Input: part model. Units: mm. Frame: model coordinates. A direction names the side the tool comes from. Give positions to 0.01 mm unless a question says otherwise; leave off trailing zeros. Loops run counter-clockwise (first coordinate to the right, second up) from the corner with the lowest first, then second, coordinate; pieces in that order, holes last. Notation, with made-up numbers: (-11, -34.5) - (44, -34.5) arc R8 cw to (44, -28.5) - close; hole circle Ø9 at (-17.5, -21.75). An arc over 180 degrees is marked (long way). Answer as a JSON object with one key per item and string values.
from build123d import *

# Parameters (mm, degrees)
F0_W     = 7.8486
F0_H     = 7.8486
F1_DEPTH = 9.6012
F2_R     = 1.7653
F3_DEPTH = 1.6256
F4_W     = 4.8514
F4_H     = 4.8514
F5_DEPTH = 8.3312


with BuildPart() as f1:
    # F0 (on Top) → F1 (new body)
    with BuildSketch(Plane.XY):
        Rectangle(F0_W, F0_H)
    extrude(amount=F1_DEPTH)

    # F2 (on face) → F3 (join)
    with BuildSketch(Plane.XY.offset(9.6012)):
        Circle(F2_R)
    extrude(amount=F3_DEPTH)

    # F4 (on face) → F5 (cut)
    with BuildSketch(Plane(origin=(0, 0, 0), x_dir=(1, 0, 0), z_dir=(0, 0, -1))):
        Rectangle(F4_W, F4_H)
    extrude(amount=-F5_DEPTH, mode=Mode.SUBTRACT)


solid = f1.part
Item 1: Cut plane D-D (x = 2). Return loops of the section in (y, z).
Geometry check:
{"outline": "(-3.92, 0) - (-2.43, 0) - (-2.43, 8.33) - (2.43, 8.33) - (2.43, 0) - (3.92, 0) - (3.92, 9.6) - (-3.92, 9.6) - close"}
Item 2: Access query for faces 1 (the face through (0, -2.426, 4)), 2 (the face through (3.924, 0, 5)). Directions: +Z, -Z, +X, -X, +Y, -Y. A direction counts if a zero-diameter tool reaches every point of the face in a straight line with its end or side. Return the directions, or none.
Geometry check:
{"face 1": "-Z", "face 2": "+Z, -Z, +X, +Y, -Y"}
Item 3: Cut plane B-B (x = 0). Return loops of the section in (y, z), then the cut area to 3 significant figures.
Geometry check:
{"outline": "(-3.92, 0) - (-2.43, 0) - (-2.43, 8.33) - (2.43, 8.33) - (2.43, 0) - (3.92, 0) - (3.92, 9.6) - (1.77, 9.6) - (1.77, 11.23) - (-1.77, 11.23) - (-1.77, 9.6) - (-3.92, 9.6) - close", "area": "40.7 mm2"}
Item 4: Mould query, pull axis Y, two halves, no side actions, for faces 3 (the face through (0, 0, 8.331)), 4 (the face through (2.426, 0, 4)), 5 (the face through (0.81, -1.57, 10.4)), 6 (the face through (-2, 0, 9.601)). Classes: released by +Y, released by -Y, zero draft, split by the parting line, or undercut.
Geometry check:
{"face 3": "undercut", "face 4": "undercut", "face 5": "split by the parting line", "face 6": "zero draft"}
Item 5: Material intervals for line 1 (Y direction, x = -1, z = 6.5); line 2 (Z direction, x = 2, y = -2), sorted ascending. Write a range as [from, to].
Geometry check:
{"line 1": "y = [-3.92, -2.43], [2.43, 3.92]", "line 2": "z = [8.33, 9.6]"}
Item 6: Cut plane A-A (z = 0.5). Return loops of the section in (x, y).
Geometry check:
{"outline": "(-3.92, -3.92) - (3.92, -3.92) - (3.92, 3.92) - (-3.92, 3.92) - close; hole (-2.43, -2.43) - (2.43, -2.43) - (2.43, 2.43) - (-2.43, 2.43) - close"}
Item 7: Contact query for a flat-ended pin moving along its axis: P1, Ø1.5, axis at x = 2, y = 0, coming from the -Z side. Output: stop coordinate, or through.
Geometry check:
{"P1": "stops at z = 0"}
